from build123d import *
from build123d.topology import SkipClean

# Parameters (mm, degrees)
BOSS_EXTRUDE1_DEPTH     = 5
CUT_EXTRUDE1_DEPTH      = 46.552167896
CUT_EXTRUDE1_DEPTH_BACK = 46.552167896
SKETCH2_R               = 0.25


with BuildPart() as part:
    # Sketch1 → Boss-Extrude1 (new body)
    with BuildSketch(Plane(origin=(0, 0, 0), x_dir=(1, 0, 0), z_dir=(0, 1, 0))):
        with BuildLine():
            Line((-40, 5), (0, 5))
            ThreePointArc((0, 5), (5, 0), (0, -5))
            Line((0, -5), (-40, -5))
            ThreePointArc((-40, -5), (-45, 0), (-40, 5))
        make_face()
    extrude(amount=BOSS_EXTRUDE1_DEPTH)

    # Sketch2 → Cut-Extrude1 (cut, two sides: drawn at the far end of the back side and taken through both)
    with SkipClean():  # the faces are left unmerged after this step: merging them gives an invalid solid
        with BuildSketch(Plane(origin=(0, 5, 0), x_dir=(1, 0, 0), z_dir=(0, 1, 0)).offset(-CUT_EXTRUDE1_DEPTH_BACK)):
            with Locations((-18.775, -1.029259443)):
                Circle(SKETCH2_R)
            with BuildLine():
                Line((-18.775, -1.029259443), (-21.225, -1.029259443))
                ThreePointArc((-21.225, -1.029259443), (-20, 1.6), (-18.775, -1.029259443))
            make_face()
            with BuildLine():
                ThreePointArc((-18.775, -1.029259443), (-20, 1.6), (-21.225, -1.029259443))
                Line((-21.225, -1.029259443), (-18.775, -1.029259443))
            make_face()
            with BuildLine():
                ThreePointArc((-18.629623366, -0.82587401), (-18.606910194, 0.786956665), (-20, 1.6))
                Line((-20, 1.6), (-20, -1.029259443))
                Line((-20, -1.029259443), (-19.025, -1.029259443))
                ThreePointArc((-19.025, -1.029259443), (-18.889358737, -0.806948671), (-18.629623366, -0.82587401))
            make_face()
            with BuildLine():
                Line((-20, -1.029259443), (-20, 1.6))
                ThreePointArc((-20, 1.6), (-21.393089806, 0.786956665), (-21.370376634, -0.82587401))
                ThreePointArc((-21.370376634, -0.82587401), (-21.110641263, -0.806948671), (-20.975, -1.029259443))
                Line((-20.975, -1.029259443), (-20, -1.029259443))
            make_face()
            with Locations((-21.225, -1.029259443)):
                Circle(SKETCH2_R)
        extrude(amount=CUT_EXTRUDE1_DEPTH + CUT_EXTRUDE1_DEPTH_BACK, mode=Mode.SUBTRACT)


solid = part.part
Source: CAD feature listing. Evaluate the final solid. Frame: model axes, mm. Round coordinates to 2 decimals unless told otherwise and drop trailing zeros. Loops run counter-clockwise (first coordinate to the right, second up) from the corner with the lowest first, then second, coordinate; pieces in that order, holes last. Notation, with made-up numbers: (72.25, 8) - (90.25, 8) arc R16 cw to (90.25, 16) - close; hole circle Ø10 at (52, -25.5). An arc over 180 degrees is marked (long way). Write item = value, one per line. Start each with the question number.
(1) Section query C-C, the plane y = 2.35. Output: boundary loops of the cut face in (x, z) (3 decimals), plus the area to 3 significant figures.
(2) Pin query (flat end, axial travel): pin 1 (1 mm diameter, centred on y = 2.5, z = -3, fed in from +X). Return the tip coordinate at first contact, or that it passes through.
(3) Section query D-D, the plane z = 3. Output: boundary loops of the cut face in (x, y), plus the area to 3 significant figures.
(4) Section query A-A, the plane x = -20. Output: boundary loops of the cut face in (y, z).
(5) Ray query, line 1 along Z through (x, y) = (-20, 3.25); line 2 along X through (y, z) = (1.5, 0); line 3 along X through (y, z) = (3.6, -0.5). Return the intervals inside material, ascending. Write a range as from..to.
(6) Section query B-B, the plane z = -0.5. Output: boundary loops of the cut face in (x, y).
(7) Pull-direction query (Z, two-part tool) for faces 1 (the face through (-20, 2, 1.029)), 2 (the face through (5, 2, 0)), 3 (the face through (-20, 2, 5)), 4 (the face through (-20, 2.5, -1.6)); classes: +Z half, -Z half, draft (parallel to the pull), parting line (faces both ways), or undercut.
Conclusion:
q1.outline = (-40, -5) - (0, -5) arc R5 ccw to (0, 5) - (-40, 5) arc R5 ccw to start; hole (-21.37, 0.826) arc R1.6 ccw (long way) to (-18.63, 0.826) arc R0.25 ccw (long way) to (-19.025, 1.029) - (-20.975, 1.029) arc R0.25 ccw (long way) to start
q1.area = 471 mm2
q2.pin_1 = 4.33
q3.outline = (-44, 0) - (4, 0) - (4, 5) - (-44, 5) - close
q3.area = 240 mm2
q4.outline = (0, -5) - (5, -5) - (5, -1.6) - (0, -1.6) - close; (0, 1.03) - (5, 1.03) - (5, 5) - (0, 5) - close
q5.line_1 = -5..-1.6, 1.03..5
q5.line_2 = -45..-21.6, -18.4..5
q5.line_3 = -44.97..-21.52, -18.48..4.97
q6.outline = (-44.97, 0) - (-21.52, 0) - (-21.52, 5) - (-44.97, 5) - close; (-18.48, 0) - (4.97, 0) - (4.97, 5) - (-18.48, 5) - close
q7.face_1 = undercut
q7.face_2 = parting line
q7.face_3 = +Z half
q7.face_4 = undercut
